Can you work these out from the model? Positions are in its coordinate system, mm. A direction names the side the tool comes from. Give positions to 0.01 mm unless a question says otherwise; leave off trailing zeros. Write each loop counter-clockwise with the first axis right and the second up, starting at its lowest first coordinate (ties: lowest second). Pieces come first, ordered by that corner, then holes. Notation, with made-up numbers: (72, 78.5) -> (112, 78.5) arc R23 cw to (112, 117.5) -> close; hole circle Ø7 at (-1.5, 71). An arc over 180 degrees is marked (long way). Answer as CSV lines item,"result". Start each with the question number.
1. I need wall thicknesses on line 1 (Z direction, x = 5, y = 8.5); line 2 (Z direction, x = 42, y = -11.5); line 3 (X direction, y = 23.5, z = 39.5). Which ranges of each line are inside material? Lowest first, please. Write a range as [from, to].
2. I'm going to push flat-ended pins straight in: P1, Ø6, axis at y = 15.5, z = -0.5, coming from the +X side; P2, Ø5, axis at y = 2.5, z = 39.5, coming from the +X side; P3, Ø2, axis at y = -17.5, z = 36, coming from the -X side. Where does each tip first touch, or does it pass through?
3. If we mould it in two halves opening along Y, with no side actions, what happens to faces 1 (the face through (0, 31.011, -1)), 2 (the face through (1, 0, -9.389)), 3 (the face through (27, 28.011, 21))? For each: pulls with the +Y half, pulls with the -Y half, needs draft (parallel to the pull), parting line crosses it, or undercut.
4. If we section it at A-A on x = 7: Write out the boundary of the cut face in (y, z), plus the area to 3 significant figures.
5. If we section it at B-B on y = 12: Write out the boundary of the cut face in (x, z).
6. If we section it at C-C on z = 11.5: Write out the boundary of the cut face in (x, y), plus the area to 3 significant figures.
7. If we section it at D-D on x = 30: Write out the boundary of the cut face in (y, z), plus the area to 3 significant figures.
8. On a 3-axis mill with a long thin cutter (end or side, diameter ignored), from which of +Z, -Z, +X, -X, +Y, -Y can I reach the whole of each face in a straight line? I mean faces 4 (the face through (-47.623, 0, -5)), 5 (the face through (26.823, -29.49, 19.822)), 6 (the face through (-27, -28.011, 21)). Say none if no direction works.
Autodesk Fusion 360 part; units mm, degrees
ref_plane "WorkPlane1" through (0, 28.011, 0) normal (0, 1, 0) x (0, 0, 1)
sketch "Sketch2" plane through (0, 28.011, 0) normal (0, 1, 0) x (1, 0, 0)
  line L0 (-47.6227, 0.6459) -> (-8.7892, -42.213)
  line L1 (-8.7892, -39.7251) -> (-48.648, 4.2654)
  line L2 (-8.7892, -42.213) -> (0, -42.213)
  line L3 (0, -42.213) -> (0, -36.199)
  line L4 (0, -36.199) -> (-8.7892, -36.199)
  line L5 (-8.7892, -36.199) -> (-8.7892, -42.213)
  line L6 (-47.6227, 0.6459) -> (0, 0.6459)
  line L7 (0, 0.6459) -> (0, 9.3893)
  line L8 (0, 9.3893) -> (-47.6227, 9.3893)
  line L9 (-47.6227, 9.3893) -> (-47.6227, 0.6459)
extrude "Extrude1" add sketch "Sketch2" along normal blind 3
extrude "Extrude2" add sketch "Sketch2" against normal up to surface (28.011 mm away) contours L1 L6 L9 | L2 L3 L4 L5 | L1 L6 L7 L8 L9
mirror "Mirror1" about plane through (0, 0, 0) normal (1, 0, 0) of bodies 1 merged
mirror "Mirror2" about plane through (0, 0, 0) normal (0, -1, 0) of bodies 1 merged
Computed values:
1,line 1,"z = [-9.39, -0.65], [36.2, 42.21]"
1,line 2,"z = [-9.39, -0.65]"
1,line 3,"x = [-8.79, 8.79]"
2,P1,"stops at x = 47.62"
2,P2,"stops at x = 8.79"
2,P3,"stops at x = -8.79"
3,face 1,"pulls with the +Y half"
3,face 2,"needs draft"
3,face 3,"undercut"
4,outline,"(-31.01, -9.39) -> (31.01, -9.39) -> (31.01, -0.65) -> (-31.01, -0.65) -> close; (-31.01, 36.2) -> (31.01, 36.2) -> (31.01, 42.21) -> (-31.01, 42.21) -> close"
4,area,"915 mm2"
5,outline,"(-47.62, -9.39) -> (47.62, -9.39) -> (47.62, -0.65) -> (-47.62, -0.65) -> close; (-8.79, 36.2) -> (8.79, 36.2) -> (8.79, 42.21) -> (-8.79, 42.21) -> close"
6,outline,"(-36.62, -31.01) -> (-34.36, -31.01) -> (-34.36, -28.01) -> (-36.62, -28.01) -> close; (-36.62, 28.01) -> (-34.36, 28.01) -> (-34.36, 31.01) -> (-36.62, 31.01) -> close; (34.36, -31.01) -> (36.62, -31.01) -> (36.62, -28.01) -> (34.36, -28.01) -> close; (34.36, 28.01) -> (36.62, 28.01) -> (36.62, 31.01) -> (34.36, 31.01) -> close"
6,area,"27.1 mm2"
7,outline,"(-31.01, -9.39) -> (31.01, -9.39) -> (31.01, -0.65) -> (-31.01, -0.65) -> close; (-31.01, 16.32) -> (-28.01, 16.32) -> (-28.01, 18.8) -> (-31.01, 18.8) -> close; (28.01, 16.32) -> (31.01, 16.32) -> (31.01, 18.8) -> (28.01, 18.8) -> close"
7,area,"557 mm2"
8,face 4,"+Z, -Z, -X, +Y, -Y"
8,face 5,"+Y, -Y"
8,face 6,"+Z, -X"
